Can you work these out from the model? Positions are in its coordinate system, mm. Round coordinates to 2 decimals unless told otherwise and drop trailing zeros. Loops run counter-clockwise (first coordinate to the right, second up) from the corner with the lowest first, then second, coordinate; pieces in that order, holes last.
(1) If I drill on line 1 along Y through (x, z) = (-29, -4.5); line 2 along Y through (x, z) = (-29, 1.75); line 3 along X through (y, z) = (-6, 0.25), over which ranges is the centre line in solid material (lowest first)?
(2) I want a section at B-B on y = -11. Write out the boundary of the cut face in (x, z).
(3) Will these pins go through, and if not, where does the flat tip stop? pin 1 Ø4 at (x, y) = (-29, 25) entering from -Z; pin 2 Ø2.5 at (x, z) = (47, 2) entering from +Y; pin 3 Ø1.5 at (x, z) = (46.5, 1.5) entering from -Y; pin 4 Ø4 at (x, y) = (-36.5, -26.5) entering from -Z.
(4) I want a section at A-A on x = -8.5. Write out the boundary of the cut face in (y, z), plus the area to 3 significant figures.
(5) I want a section at D-D on z = -2.5. Write out the boundary of the cut face in (x, y).
(6) I want a section at C-C on x = 36.5. Write out the boundary of the cut face in (y, z).
from build123d import *

# Parameters (mm, degrees)
SKETCH1_W           = 81
SKETCH1_H           = 61
SKETCH1_W_2         = 69
SKETCH1_H_2         = 49
EXTRUDE_THIN1_DEPTH = 3
SKETCH2_R           = 1.6
CUT_EXTRUDE1_DEPTH  = 3
FILLET1_R           = 3
SKETCH4_R           = 3
BOSS_EXTRUDE1_DEPTH = 10
BOSS_EXTRUDE2_DEPTH = 3
SKETCH5_R           = 1.25
CUT_EXTRUDE2_DEPTH  = 10
RIB2_REACH          = 79.06
SKETCH7_WALL_W      = 166.153683654
SKETCH7_WALL_H      = 2
LPATTERN1_COUNT     = 2
LPATTERN1_PITCH     = 50


with BuildPart() as part:
    # Sketch1 → Extrude-Thin1 (new body)
    with BuildSketch(Plane.XY):
        Rectangle(SKETCH1_W, SKETCH1_H)
        Rectangle(SKETCH1_W_2, SKETCH1_H_2, mode=Mode.SUBTRACT)
    extrude(amount=EXTRUDE_THIN1_DEPTH)

    # Sketch2 → Cut-Extrude1 (cut)
    with BuildSketch(Plane.XY.offset(3)):
        with Locations((-36.5, 26.5)):
            Circle(SKETCH2_R)
        with Locations((36.5, 26.5)):
            Circle(SKETCH2_R)
        with Locations((36.5, -26.5)):
            Circle(SKETCH2_R)
        with Locations((-36.5, -26.5)):
            Circle(SKETCH2_R)
    extrude(amount=-CUT_EXTRUDE1_DEPTH, mode=Mode.SUBTRACT)

    # Fillet1
    fillet1_edges = [part.edges().sort_by_distance(p)[0] for p in [
        (-34.5, 24.5, 1.5),
        (-34.5, -24.5, 1.5),
        (34.5, -24.5, 1.5),
        (34.5, 24.5, 1.5),
        (-40.5, 30.5, 1.5),
        (40.5, 30.5, 1.5),
        (40.5, -30.5, 1.5),
        (-40.5, -30.5, 1.5),
    ]]
    fillet(fillet1_edges, radius=FILLET1_R)

    # Sketch4 → Boss-Extrude1 (add)
    with BuildSketch(Plane.XY.offset(3)):
        with Locations((-29, 25)):
            Circle(SKETCH4_R)
        with Locations((50, 25)):
            Circle(SKETCH4_R)
        with Locations((50, -25)):
            Circle(SKETCH4_R)
        with Locations((-29, -25)):
            Circle(SKETCH4_R)
    extrude(amount=-BOSS_EXTRUDE1_DEPTH)


with BuildPart() as boss_extrude1_piece_1:
    # of the separate pieces the step leaves, piece 1, a body of its own (boss_extrude1_pieces)
    add(part.part.solids().sort_by_distance((-37.5, -30.5, 0))[0])



with BuildPart() as boss_extrude1_piece_2:
    # of the separate pieces the step leaves, piece 2, a body of its own (boss_extrude1_pieces)
    add(part.part.solids().sort_by_distance((53, 25, 3))[0])


with BuildPart() as boss_extrude1_piece_3:
    # of the separate pieces the step leaves, piece 3, a body of its own (boss_extrude1_pieces)
    add(part.part.solids().sort_by_distance((53, -25, 3))[0])


with BuildPart() as boss_extrude1_piece_1_1:
    add(boss_extrude1_piece_1.part)

    add(boss_extrude1_piece_2.part)  # Boss-Extrude2 merges Boss-Extrude1 piece 2

    add(boss_extrude1_piece_3.part)  # Boss-Extrude2 merges Boss-Extrude1 piece 3
    # Sketch6 → Boss-Extrude2 (add)
    with BuildSketch(Plane.XY.offset(3)):
        with BuildLine():
            Line((50, 28), (40.458039892, 28))
            Line((40.458039892, 28), (40.5, 22))
            Line((40.5, 22), (50, 22))
            ThreePointArc((50, 22), (53, 25), (50, 28))
        make_face()
        with BuildLine():
            Line((40.5, -22), (40.458039892, -28))
            Line((40.458039892, -28), (50, -28))
            ThreePointArc((50, -28), (53, -25), (50, -22))
            Line((50, -22), (40.5, -22))
        make_face()
    extrude(amount=-BOSS_EXTRUDE2_DEPTH)

    # Sketch5 → Cut-Extrude2 (cut)
    with BuildSketch(Plane(origin=(0, 0, -7), x_dir=(-1, 0, 0), z_dir=(0, 0, -1))):
        with Locations((-50, 25)):
            Circle(SKETCH5_R)
        with Locations((29, 25)):
            Circle(SKETCH5_R)
        with Locations((-50, -25)):
            Circle(SKETCH5_R)
        with Locations((29, -25)):
            Circle(SKETCH5_R)
    extrude(amount=-CUT_EXTRUDE2_DEPTH, mode=Mode.SUBTRACT)

    # Sketch7 wall → Rib2 (add, up to next)
    with BuildSketch(Plane(origin=(44.051757722, 25, -3.500496738), x_dir=(-0.716336631923, 0, 0.697754849331), z_dir=(0.697754849331, 0, 0.716336631923)), mode=Mode.PRIVATE) as rib2_sk1:
        Rectangle(SKETCH7_WALL_W, SKETCH7_WALL_H)
    rib2_tool1 = extrude(rib2_sk1.sketch, amount=RIB2_REACH, mode=Mode.PRIVATE) - boss_extrude1_piece_1_1.part
    rib2 = rib2_tool1.solids().sort_by_distance((44.051757722, 25, -3.500496738))[0]
    add(rib2)

    # LPattern1: Rib2 ×2
    with Locations(*[(0, -i * LPATTERN1_PITCH, 0) for i in range(1, LPATTERN1_COUNT)]):
        add(rib2)


solid = boss_extrude1_piece_1_1.part
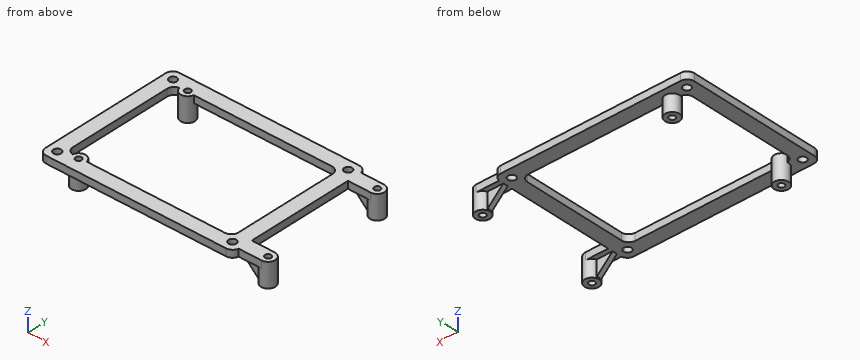
Filled sheet:
1. line 1: y = -28 to -26.25, -23.75 to -22, 22 to 23.75, 26.25 to 28
1. line 2: y = -30.5 to -26.25, -23.75 to -22, 22 to 23.75, 26.25 to 30.5
1. line 3: x = -40.5 to -34.5, 34.5 to 40.5
2. outline: (-40.5, 0) - (-34.5, 0) - (-34.5, 3) - (-40.5, 3) - close; (34.5, 0) - (40.5, 0) - (40.5, 3) - (34.5, 3) - close
3. pin 1: stops at z = -7
3. pin 2: stops at y = 28
3. pin 3: stops at y = -28
3. pin 4: stops at z = 0
4. outline: (-30.5, 0) - (-24.5, 0) - (-24.5, 3) - (-30.5, 3) - close; (24.5, 0) - (30.5, 0) - (30.5, 3) - (24.5, 3) - close
4. area: 36.0 mm2
5. outline: circle Ø6 at (-29, -25); circle Ø6 at (-29, 25); (43.02, -26) - (47.17, -26) arc R3 ccw (long way) to (47.17, -24) - (43.02, -24) - close; (43.02, 24) - (47.17, 24) arc R3 ccw (long way) to (47.17, 26) - (43.02, 26) - close; hole circle Ø2.5 at (-29, -25); hole circle Ø2.5 at (-29, 25); hole circle Ø2.5 at (50, -25); hole circle Ø2.5 at (50, 25)
6. outline: (-30.5, 0) - (-28.1, 0) - (-28.1, 3) - (-30.5, 3) - close; (-24.9, 0) - (24.9, 0) - (24.9, 3) - (-24.9, 3) - close; (28.1, 0) - (30.5, 0) - (30.5, 3) - (28.1, 3) - close
